from build123d import *

# Parameters (mm, degrees)
SKETCH1_R                      = 40
SKETCH1_W                      = 45
SKETCH1_H                      = 45
BOSS_EXTRUDE1_DEPTH            = 60
BOSS_EXTRUDE2_START            = 40
SKETCH2_R                      = 40
SKETCH2_W                      = 45
SKETCH2_H                      = 45
BOSS_EXTRUDE2_DEPTH            = 40
BOSS_EXTRUDE3_START            = 60
BOSS_EXTRUDE3_DEPTH            = 60
FILLET1_R                      = 5
SKETCH7_W                      = 55
SKETCH7_H                      = 20
CUT_EXTRUDE4_DEPTH             = 10
CUT_EXTRUDE5_DEPTH             = 29
F_3_0MM_DOWEL_HOLE2_D          = 3
F_3_0MM_DOWEL_HOLE2_DEPTH      = 5
F_3_0MM_DOWEL_HOLE2_TIP        = 0.901290929
CUT_EXTRUDE6_REACH             = 134.665
CUT_EXTRUDE6_DIRECTION_2_REACH = 134.665


with BuildPart() as part:
    # Sketch1 → Boss-Extrude1 (new body)
    with BuildSketch(Plane.XY):
        Circle(SKETCH1_R)
        Rectangle(SKETCH1_W, SKETCH1_H, mode=Mode.SUBTRACT)
    extrude(amount=BOSS_EXTRUDE1_DEPTH)

    # Sketch2 → Boss-Extrude2 (add)
    # profile 1 of 2: a face of its own
    with BuildSketch(Plane(origin=(0, 0, 0), x_dir=(-1, 0, 0), z_dir=(0, 0, -1)).offset(BOSS_EXTRUDE2_START)):
        Circle(SKETCH2_R)
        Rectangle(SKETCH2_W, SKETCH2_H, mode=Mode.SUBTRACT)
    # profile 2 of 2: a face of its own
    with BuildSketch(Plane(origin=(0, 0, 0), x_dir=(-1, 0, 0), z_dir=(0, 0, -1)).offset(BOSS_EXTRUDE2_START)):
        Rectangle(SKETCH2_W, SKETCH2_H)
    extrude(amount=-BOSS_EXTRUDE2_DEPTH)

    # Sketch3 → Boss-Extrude3 (add)
    with BuildSketch(Plane(origin=(0, 0, -40), x_dir=(-1, 0, 0), z_dir=(0, 0, -1)).offset(BOSS_EXTRUDE3_START)):
        with BuildLine():
            Line((-10, -38.729833462), (-10, 38.729833462))
            ThreePointArc((-10, 38.729833462), (-40, 0), (-10, -38.729833462))
        make_face()
    extrude(amount=-BOSS_EXTRUDE3_DEPTH)

    # Fillet1
    fillet1_edges = [part.edges().sort_by_distance(p)[0] for p in [
        (-22.5, 22.5, 30),
        (-22.5, -22.5, 30),
        (22.5, -22.5, 30),
        (22.5, 22.5, 30),
        (22.5, 0, 60),
        (0, -22.5, 60),
        (-22.5, 0, 60),
        (0, 22.5, 60),
        (0, -22.5, 0),
    ]]
    fillet(fillet1_edges, radius=FILLET1_R)

    # Sketch7 → Cut-Extrude4 (cut)
    with BuildSketch(Plane.ZY.offset(-10)):
        with Locations((-70, 0)):
            Rectangle(SKETCH7_W, SKETCH7_H)
    extrude(amount=-CUT_EXTRUDE4_DEPTH, mode=Mode.SUBTRACT)

    # Sketch8 → Cut-Extrude5 (cut)
    with BuildSketch(Plane.ZY.offset(-20)):
        Polygon((-50, 10), (-90, 10), (-90, 0), (-90, -10), (-50, -10), (-50, 0), align=None)
    extrude(amount=-CUT_EXTRUDE5_DEPTH, mode=Mode.SUBTRACT)

    # 3.0mm Dowel Hole2
    with Locations(Plane.ZY.offset(-20)):
        with Locations((-46, 5), (-94, 5), (-94, -5), (-46, -5)):
            Hole(F_3_0MM_DOWEL_HOLE2_D / 2, depth=F_3_0MM_DOWEL_HOLE2_DEPTH)
            with Locations((0, 0, -(F_3_0MM_DOWEL_HOLE2_DEPTH + F_3_0MM_DOWEL_HOLE2_TIP / 2))):  # 118° drill point
                Cone(0, F_3_0MM_DOWEL_HOLE2_D / 2, F_3_0MM_DOWEL_HOLE2_TIP, mode=Mode.SUBTRACT)

    # Cut-Extrude6: up to this face of the body (flat: up to its plane)
    cut_extrude6_end = Plane(part.part.faces().sort_by_distance((15, 0, -42.5))[0])
    # Sketch18 → Cut-Extrude6 (cut, up to the picked face)
    with BuildSketch(Plane(origin=(0, 0, -60), x_dir=(-1, 0, 0), z_dir=(0, 0, -1)), mode=Mode.PRIVATE) as cut_extrude6_sk1:
        with BuildLine():
            Line((-25, -10), (-25, 10))
            Line((-25, 10), (-38.729833462, 10))
            ThreePointArc((-38.729833462, 10), (-40, 0), (-38.729833462, -10))
            Line((-38.729833462, -10), (-25, -10))
        make_face()
    cut_extrude6_tool1 = split(extrude(cut_extrude6_sk1.sketch, amount=-CUT_EXTRUDE6_REACH, mode=Mode.PRIVATE), bisect_by=cut_extrude6_end, keep=Keep.BOTH, mode=Mode.PRIVATE)
    add(cut_extrude6_tool1.solids().sort_by(Axis((32.294564, 0, -60), (0, 0, 1)))[0], mode=Mode.SUBTRACT)

    # Cut-Extrude6 direction 2: up to this face of the body (flat: up to its plane)
    cut_extrude6_direction_2_end = Plane(part.part.faces().sort_by_distance((15, 0, -97.5))[0])
    # Sketch18 → Cut-Extrude6 direction 2 (cut, up to the picked face)
    with BuildSketch(Plane(origin=(0, 0, -60), x_dir=(-1, 0, 0), z_dir=(0, 0, -1)), mode=Mode.PRIVATE) as cut_extrude6_direction_2_sk1:
        with BuildLine():
            Line((-25, -10), (-25, 10))
            Line((-25, 10), (-38.729833462, 10))
            ThreePointArc((-38.729833462, 10), (-40, 0), (-38.729833462, -10))
            Line((-38.729833462, -10), (-25, -10))
        make_face()
    cut_extrude6_direction_2_tool1 = split(extrude(cut_extrude6_direction_2_sk1.sketch, amount=CUT_EXTRUDE6_DIRECTION_2_REACH, mode=Mode.PRIVATE), bisect_by=cut_extrude6_direction_2_end, keep=Keep.BOTH, mode=Mode.PRIVATE)
    add(cut_extrude6_direction_2_tool1.solids().sort_by(Axis((32.294564, 0, -60), (0, 0, -1)))[0], mode=Mode.SUBTRACT)


solid = part.part
Read the model definition and answer for the solid it produces. Units are mm, in the model's axes. A direction names the side the tool comes from. Give positions to 0.01 mm unless a question says otherwise; leave off trailing zeros. Write each loop counter-clockwise with the first axis right and the second up, starting at its lowest first coordinate (ties: lowest second). Pieces come first, ordered by that corner, then holes. Notation, with made-up numbers: (71.5, 43.5) - (89.5, 43.5) arc R23 cw to (89.5, 52.5) - close; hole circle Ø1 at (-25.5, 47.5). An arc over 180 degrees is marked (long way). Answer in a Markdown table with one row per item. Add a question column.
Item 1: A tool of negligible diameter and unlimited length cuts with its end or side. For faces 4 (the face through (25, 0, -94)), 5 (the face through (21, 21.07, 27.88)), 6 (the face through (22, 0, -90)), 7 (the face through (20, 0, -46)), 8 (the face through (10, 17, -70)), from which of +Z, -Z, +X, -X, +Y, -Y can it reach the whole face along a straight path? Write none if from no direction.
Item 2: Section D-D, the plane x = 30.5 is taken. Write down the section's boundary in (y, z), and give its area (3 significant figures).
Item 3: Section C-C, the plane x = 0 is taken. Write down the section's boundary in (y, z).
Item 4: Determine the mould class of faces 1 (the face through (22.54, 5.07, -44.5)), 2 (the face through (0, -22.5, 30)), 3 (the face through (3, -29, 60)) for opening direction Y: pulls with the +Y half, pulls with the -Y half, needs draft (parallel to the pull), parting line crosses it, or undercut.
Item 5: Find the intervals of material crossed by L1, parallel to Z at x = 21, y = 5; L2, parallel to X at y = -10, z = 4.5; L3, parallel to Z at x = 13.5, y = 5, in increasing order.
Item 6: Flat-ended cylindrical pins translate along their axes: P1, Ø8, axis at y = -0.5, z = -47, coming from the +X side; P2, Ø3, axis at y = 25, z = 30.5, coming from the -X side; P3, Ø5, axis at y = 5, z = -94, coming from the -X side; P4, Ø10, axis at x = 3, z = -82, coming from the -Y side (3 decimals). Find the tip coordinate at first contact, or state that the pin passes through.
Item 7: Section B-B, the plane y = 32 is taken. Write down the section's boundary in (x, z).
Item 8: Section A-A, the plane z = -58 is taken. Write down the section's boundary in (x, y).
Recorded:
| question | item | result |
|---|---|---|
| 1 | face 4 | +X |
| 1 | face 5 | +Z |
| 1 | face 6 | +X, -X |
| 1 | face 7 | -X |
| 1 | face 8 | -Z, -X, +Y, -Y |
| 2 | outline | (-25.88, -100) - (25.88, -100) - (25.88, 60) - (-25.88, 60) - close; hole (-10, -97.5) - (10, -97.5) - (10, -42.5) - (-10, -42.5) - close |
| 2 | area | 7,180 mm2 |
| 3 | outline | (-40, -40) - (40, -40) - (40, 60) - (27.5, 60) arc R5 ccw to (22.5, 55) - (22.5, 0) - (-17.5, 0) arc R5 cw to (-22.5, 5) - (-22.5, 55) arc R5 ccw to (-27.5, 60) - (-40, 60) - close |
| 4 | face 1 | undercut |
| 4 | face 2 | undercut |
| 4 | face 3 | needs draft |
| 5 | L1 | z = -100 to -95.5, -92.5 to -90, -50 to -47.5, -44.5 to 0 |
| 5 | L2 | x = -38.73 to -22.5, 22.5 to 38.73 |
| 5 | L3 | z = -100 to -97.5, -42.5 to 0 |
| 6 | P1 | stops at x = 25 |
| 6 | P2 | stops at x = -32.37 |
| 6 | P3 | stops at x = 20 |
| 6 | P4 | passes through |
| 7 | outline | (-24, -40) - (10, -40) - (10, -100) - (24, -100) - (24, 60) - (-24, 60) - close |
| 8 | outline | (10, -38.73) arc R40 ccw to (38.73, -10) - (10, -10) - close; (10, 10) - (38.73, 10) arc R40 ccw to (10, 38.73) - close |
